Verification items for the finished model (mm, model axes). A direction names the side the tool comes from. Coordinates: 2 decimals unless noted, no trailing zeros. Write each loop counter-clockwise with the first axis right and the second up, starting at its lowest first coordinate (ties: lowest second). Pieces come first, ordered by that corner, then holes. Notation, with made-up numbers: (88.5, 30.5) -> (143.5, 30.5) arc R17 ccw to (143.5, 50.5) -> close; hole circle Ø7 at (85.25, -25). An arc over 180 degrees is marked (long way). Answer in a Markdown table with one row per item.
Autodesk Inventor part; units mm, degrees
ref_plane "YZ Plane" through (0, 0, 0) normal (1, 0, 0) x (0, 1, 0)
ref_plane "XZ Plane" through (0, 0, 0) normal (0, 1, 0) x (-1, 0, 0)
ref_plane "XY Plane" through (0, 0, 0) normal (0, 0, 1) x (1, 0, 0)
sketch "Sketch1" plane through (0, 0, 0) normal (0, 1, 0) x (-1, 0, 0)
  circle A0 centre (-30, -5.1319) radius 1.5
  arc A1 (-31.1155, 2.2846) -> (-30, -12.6319) centre (-30, -5.1319) ccw
  arc A2 (-30, -12.6319) -> (-31.1155, 2.2846) centre (-30, -5.1319) ccw construction
  circle A3 centre (-16.9706, -0.5878) radius 1.5
  circle A4 centre (16.9706, -0.5878) radius 1.5
  circle A5 centre (16.9706, -0.5878) radius 5 construction
  line L0 (-16.9706, 4.4122) -> (-31.1155, 2.2846)
  circle A6 centre (-16.9706, -0.5878) radius 5 construction
  circle A7 centre (-7.8058, -8.4213) radius 1.55
  line L1 (0, -8.4213) -> (-15.6117, -8.4213) construction
  circle A8 centre (0, 0) radius 1.55
  line L2 (-16.9706, 4.4122) -> (16.9706, 4.4122)
  line L3 (30, -12.6319) -> (-30, -12.6319)
  circle A9 centre (30, -5.1319) radius 1.5
  line L4 (0, 4.2106) -> (0, -4.2106) construction
  line L5 (0, -4.2106) -> (0, -12.6319) construction
  line L6 (0, -4.2106) -> (3.1574, -4.2106) construction
  line L7 (0, -8.4213) -> (15.6117, -8.4213) construction
  line L8 (16.9706, 4.4122) -> (31.1155, 2.2846)
  arc A10 (31.1155, 2.2846) -> (30, -12.6319) centre (30, -5.1319) ccw construction
  arc A11 (30, -12.6319) -> (31.1155, 2.2846) centre (30, -5.1319) ccw
  circle A12 centre (7.8058, -8.4213) radius 1.55
  point P0 (0, 0)
  point P1 (0, 0)
  dimension "d0" = 10
  dimension "d1" = 10
  dimension "d2" = 15
  dimension "d3" = 15
  dimension "d4" = 3.1
  dimension "d5" = 3.1
  dimension "d6" = 3.1
sketch "Sketch2" plane through (0, 0, 0) normal (0, 1, 0) x (-1, 0, 0)
  circle A0 centre (15, 9.8681) radius 3
  circle A1 centre (16.9706, -0.5878) radius 1.5
  arc A2 (3.1574, 6.6664) -> (-3.1574, 6.6664) centre (0, 4.2106) ccw
  line L0 (3.1574, 6.6664) -> (11.0366, -3.464)
  arc A3 (11.0366, -3.464) -> (13.9152, -6.7248) centre (38.6639, 18.024) ccw
  line L1 (13.9152, -6.7248) -> (21.1612, -13.9708)
  arc A4 (30.0072, 37.5736) -> (30.286, 34.6489) centre (32.7505, 36.3595) ccw
  arc A5 (35.8309, 43.8114) -> (30.0072, 37.5736) centre (41.895, 32.3124) ccw
  circle A6 centre (25.4558, 41.8386) radius 1.5
  circle A7 centre (30, 54.8681) radius 1.5
  circle A8 centre (16.9706, 50.3239) radius 1.5
  circle A9 centre (15, 39.8681) radius 3
  circle A10 centre (24.2029, 72.4055) radius 1.5
  line L2 (27.7949, 74.3102) -> (17.0958, 107.9924)
  arc A11 (17.0958, 107.9924) -> (14.6505, 110.5406) centre (13.2835, 106.7814) ccw
  circle A12 centre (13.2835, 106.7814) radius 1.5
  line L3 (14.6505, 110.5406) -> (2.0505, 115.1224)
  circle A13 centre (-24.2029, 72.4055) radius 1.5
  arc A14 (2.0505, 115.1224) -> (-2.0505, 115.1224) centre (0, 109.4837) ccw
  line L4 (-17.0958, 107.9924) -> (-27.7949, 74.3102)
  circle A15 centre (-13.2835, 106.7814) radius 1.5
  arc A16 (-14.6505, 110.5406) -> (-17.0958, 107.9924) centre (-13.2835, 106.7814) ccw
  line L5 (-2.0505, 115.1224) -> (-14.6505, 110.5406)
  line L6 (-25.5, 17.3681) -> (-25.5, 32.3681)
  line L7 (-28.5, 32.3681) -> (-28.5, 17.3681)
  line L8 (-31, 32.3681) -> (-31, 17.3681)
  arc A17 (-28.5, 17.3681) -> (-25.5, 17.3681) centre (-27, 17.3681) ccw
  arc A18 (-31, 17.3681) -> (-30.286, 15.0873) centre (-27, 17.3681) ccw
  arc A19 (-30.0072, 37.5736) -> (-35.8309, 43.8114) centre (-41.895, 32.3124) ccw
  arc A20 (-25.5, 32.3681) -> (-28.5, 32.3681) centre (-27, 32.3681) ccw
  arc A21 (-30.286, 34.6489) -> (-31, 32.3681) centre (-27, 32.3681) ccw
  arc A22 (-30.286, 34.6489) -> (-30.0072, 37.5736) centre (-32.7505, 36.3595) ccw
  circle A23 centre (-25.4558, 41.8386) radius 1.5
  circle A24 centre (-15, 39.8681) radius 3
  circle A25 centre (-16.9706, 50.3239) radius 1.5
  arc A26 (-30.0072, 12.1625) -> (-30.286, 15.0873) centre (-32.7505, 13.3766) ccw
  arc A27 (-35.8309, 5.9248) -> (-30.0072, 12.1625) centre (-41.895, 17.4238) ccw
  arc A28 (-35.8309, 5.9248) -> (-21.1612, -13.9708) centre (-30, -5.1319) ccw
  line L9 (-21.1612, -13.9708) -> (-13.9152, -6.7248)
  circle A29 centre (-15, 9.8681) radius 3
  circle A30 centre (-25.4558, 7.8975) radius 1.5
  circle A31 centre (-16.9706, -0.5878) radius 1.5
  circle A32 centre (-30, -5.1319) radius 1.5
  line L10 (-11.0366, -3.464) -> (-3.1574, 6.6664)
  arc A33 (-13.9152, -6.7248) -> (-11.0366, -3.464) centre (-38.6639, 18.024) ccw
  line L11 (31, 17.3681) -> (31, 32.3681)
  arc A34 (28.5, 32.3681) -> (25.5, 32.3681) centre (27, 32.3681) ccw
  line L12 (25.5, 32.3681) -> (25.5, 17.3681)
  line L13 (28.5, 17.3681) -> (28.5, 32.3681)
  arc A35 (31, 32.3681) -> (30.286, 34.6489) centre (27, 32.3681) ccw
  arc A36 (-34.9925, 66.3278) -> (-27.7949, 74.3102) centre (-40.1848, 78.2458) ccw
  arc A37 (-34.9925, 66.3278) -> (-35.8309, 43.8114) centre (-30, 54.8681) ccw
  circle A38 centre (-30, 54.8681) radius 1.5
  arc A39 (30.0072, 12.1625) -> (35.8309, 5.9248) centre (41.895, 17.4238) ccw
  circle A40 centre (30, -5.1319) radius 1.5
  arc A41 (21.1612, -13.9708) -> (35.8309, 5.9248) centre (30, -5.1319) ccw
  circle A42 centre (25.4558, 7.8975) radius 1.5
  arc A43 (25.5, 17.3681) -> (28.5, 17.3681) centre (27, 17.3681) ccw
  arc A44 (30.286, 15.0873) -> (30.0072, 12.1625) centre (32.7505, 13.3766) ccw
  arc A45 (30.286, 15.0873) -> (31, 17.3681) centre (27, 17.3681) ccw
  arc A46 (35.8309, 43.8114) -> (34.9925, 66.3278) centre (30, 54.8681) ccw
  arc A47 (27.7949, 74.3102) -> (34.9925, 66.3278) centre (40.1848, 78.2458) ccw
  circle A48 centre (-30, -5.1319) radius 1.5 construction
  point P0 (0, 0)
  point P1 (0, 109.4837)
sketch "Sketch3" plane through (0, 0, 0) normal (0, 1, 0) x (-1, 0, 0)
  arc A0 (3.1574, 6.6664) -> (-3.1574, 6.6664) centre (0, 4.2106) ccw
  line L0 (-11.0366, -3.464) -> (-3.1574, 6.6664)
  line L1 (3.1574, 6.6664) -> (11.0366, -3.464)
  arc A1 (11.0366, -3.464) -> (13.9152, -6.7248) centre (38.6639, 18.024) ccw
  arc A2 (-13.9152, -6.7248) -> (-11.0366, -3.464) centre (-38.6639, 18.024) ccw
  line L2 (-21.1612, -13.9708) -> (-13.9152, -6.7248)
  line L3 (13.9152, -6.7248) -> (21.1612, -13.9708)
  line L4 (30, -12.6319) -> (-30, -12.6319)
  circle A3 centre (-7.8058, -8.4213) radius 1.55 construction
  circle A4 centre (7.8058, -8.4213) radius 1.55 construction
  circle A5 centre (0, 0) radius 1.55
  circle A6 centre (-16.9706, -0.5878) radius 1.5 construction
  circle A7 centre (16.9706, -0.5878) radius 1.5 construction
  line L5 (-16.9706, -2.0878) -> (16.9706, -2.0878) construction
  line L6 (7.8058, -12.6319) -> (7.8058, -2.0878) construction
  line L7 (-7.8058, -12.6319) -> (-7.8058, -2.0878) construction
  circle A8 centre (-7.8058, -7.3599) radius 1.5
  circle A9 centre (7.8058, -7.3599) radius 1.5
  line L8 (-5.032, -12.6319) -> (-5.032, -2.0878) construction
  line L9 (-5.032, -7.3599) -> (-10.6888, -7.3599) construction
  point P0 (0, 0)
  point P1 (-19.8223, -12.6319)
  point P2 (19.8223, -12.6319)
  dimension "d38" = 3
  dimension "d39" = 3
  dimension "d42" = 10.5442
extrude "Extrusion1" add sketch "Sketch3" along normal blind 6 contours L1 A1 L3 L4 L2 A2 L0 A0 | A8 | A9
sketch "Sketch4" plane through (19.8223, 0, -12.6319) normal (0, 0, -1) x (-1, 0, 0)
  line L0 (0, 0) -> (39.6447, 0)
  line L1 (39.6447, 0) -> (39.6447, 6)
  line L2 (0, 6) -> (39.6447, 6)
  line L3 (0, 0) -> (0, 6)
  point P0 (19.8223, 0)
extrude "Extrusion2" add sketch "Sketch4" along normal blind 8.5
sketch "Sketch5" plane through (0, 0, 0) normal (0, -1, 0) x (1, 0, 0)
  line L0 (-19.8223, -21.1319) -> (19.8223, -21.1319)
  line L1 (19.8223, -21.1319) -> (19.8223, -13.6319)
  line L2 (19.8223, -12.6319) -> (19.8223, -21.1319)
  line L3 (19.8223, -13.6319) -> (-19.8223, -13.6319)
  line L4 (-19.8223, -12.6319) -> (-19.8223, -21.1319)
  line L5 (-19.8223, -13.6319) -> (-19.8223, -21.1319)
  line L6 (-19.8223, -21.1319) -> (19.8223, -21.1319)
  point P0 (0, 0)
  dimension "d11" = 7.5
extrude "Extrusion3" add sketch "Sketch5" along normal blind 7
sketch "Sketch6" plane through (19.8223, 6, -12.6319) normal (1, 0, 0) x (0, 0, -1)
  line L0 (0, -6) -> (0, 0) construction
  line L1 (0, -6) -> (0, -11.9599) construction
  line L2 (0, -11.9599) -> (3.918, -11.9599) construction
  circle A0 centre (3.918, -11.9599) radius 2.55
  circle A1 centre (3.918, -11.9599) radius 4.5
  line L3 (1, -6) -> (1, -13) construction
  line L4 (1, -6) -> (1, -7) construction
  line L5 (1, -7) -> (-0.2839, -10.3492)
  line L6 (1, -7) -> (1, -8.5343)
  line L7 (1, -6) -> (1, -13)
  point P0 (-12.6319, -6)
  dimension "d15" = 5.96
  dimension "d16" = 3.918
  dimension "d17" = 5.1
  dimension "d18" = 9
  dimension "d20" = 1
fillet "Fillet2" radius 1 1 edges at (0, 0, -13.6319)
extrude "Extrusion4" add sketch "Sketch6" against normal up to surface (39.6447 mm away) contours A1
extrude "Extrusion5" cut sketch "Sketch6" against normal up to surface (39.6447 mm away) contours A0
fillet "Fillet3" radius 3 1 edges at (0, -7, -21.1319)
extrude "Extrusion6" add sketch "Sketch6" against normal up to surface (39.6447 mm away) contours A1 L5 L6
sketch "Sketch7" plane through (0, 6, 0) normal (0, 1, 0) x (1, 0, 0)
  line L0 (-19.8223, 12.6319) -> (-13.9152, 6.7248)
  arc A0 (-11.0366, 3.464) -> (-13.9152, 6.7248) centre (-38.6639, -18.024) ccw
  line L1 (-11.0366, 3.464) -> (-3.1574, -6.6664)
  arc A1 (-3.1574, -6.6664) -> (3.1574, -6.6664) centre (0, -4.2106) ccw
  line L2 (3.1574, -6.6664) -> (11.0366, 3.464)
  arc A2 (13.9152, 6.7248) -> (11.0366, 3.464) centre (38.6639, -18.024) ccw
  line L3 (13.9152, 6.7248) -> (19.8223, 12.6319)
  line L4 (19.8223, 12.6319) -> (19.8223, 21.1319)
  line L5 (-19.8223, 21.1319) -> (19.8223, 21.1319)
  line L6 (-19.8223, 12.6319) -> (-19.8223, 21.1319)
  circle A3 centre (0, 0) radius 1.55
  point P0 (0, 0)
extrude "Extrusion7" add sketch "Sketch7" along normal blind 6
fillet "Fillet4" radius 8 1 edges at (0, 12, -21.1319)
sketch "Sketch8" plane through (0, 12, 0) normal (0, 1, 0) x (1, 0, 0)
  line L0 (0, 0) -> (0, 27.291) construction
  line L1 (-0.7613, 27.291) -> (-17.5, 27.291) construction
  line L2 (0.7613, 27.291) -> (17.5, 27.291) construction
  line L3 (-17.5, 27.291) -> (-17.5, 7.1815)
  line L4 (17.5, 27.291) -> (17.5, 7.1815)
  line L5 (17.5, 7.1815) -> (23.8846, 7.1815)
  line L6 (23.8846, 7.1815) -> (23.8846, 23.5209)
  line L7 (-17.5, 7.1815) -> (-22.9652, 7.1815)
  line L8 (-22.9652, 7.1815) -> (-22.9652, 23.5209)
  line L9 (-22.9652, 23.5209) -> (23.8846, 23.5209)
  point P0 (17.5, 23.5209)
  point P1 (-17.5, 23.5209)
  dimension "d34" = 35
extrude "Extrusion8" cut sketch "Sketch8" against normal through all
sketch "Sketch9" plane through (0, 0, 0) normal (0, -1, 0) x (1, 0, 0)
  circle A0 centre (0, 0) radius 1.55
  circle A1 centre (-16.9706, -0.5878) radius 1.5
  circle A2 centre (16.9706, -0.5878) radius 1.5
  line L0 (-16.9706, -2.0878) -> (16.9706, -2.0878)
  line L1 (16.9706, -2.0878) -> (16.9706, 15.9474)
  line L2 (16.9706, 15.9474) -> (-16.9706, 15.341)
  line L3 (-16.9706, 15.341) -> (-16.9706, -2.0878)
  point P0 (0, 0)
  point P1 (-16.9706, 0.9122)
  point P2 (16.9706, 0.9122)
extrude "Extrusion9" cut sketch "Sketch9" against normal up to surface (12 mm away) contours A1 L3 L2 L1 A2 L0
fillet "Fillet5" radius 8 2 edges at (-9.9662, 6, -2.0878) (9.9662, 6, -2.0878)
extrude "Extrusion10" cut sketch "Sketch3" along normal up to surface (12 mm away) contours A8 | A9
properties part number "prig to kauri conversion front link"
1. Sectioned sample at C-C, the plane x = 14.5. Record the cut outline in (y, z).
Findings below:
| item | result |
|---|---|
| outline | (-7, -20.93) arc R3 ccw to (-5.91, -21.13) -> (4, -21.13) arc R8 ccw to (12, -13.13) -> (12, -7.31) -> (0, -7.31) -> (0, -12.63) arc R1 cw to (-1, -13.63) -> (-4.35, -12.35) arc R4.5 ccw (long way) to start; hole circle Ø5.1 at (-5.96, -16.55) |
2. Access from +Z, -Z, +X, -X, +Y, -Y to the whole of each face (thin tool, end or side, straight path). Record for faces 1 (the face through (0.25, -5.19, -18.98)), 2 (the face through (0.25, -2.65, -13)).
Findings below:
| item | result |
|---|---|
| face 1 | +X, -X |
| face 2 | +Z, +X, -X |
3. Sectioned sample at B-B, the plane z = -18. Record the cut outline in (x, y).
Findings below:
| item | result |
|---|---|
| outline | (-17.5, -10.22) -> (17.5, -10.22) -> (17.5, -8.06) -> (-17.5, -8.06) -> close; (-17.5, -3.86) -> (17.5, -3.86) -> (17.5, 10.35) -> (-17.5, 10.35) -> close |
4. Sectioned sample at D-D, the plane x = 7. Count the separate pieces of the cut face and the enclosed holes in it, and give its area (3 significant figures).
Findings below:
| item | result |
|---|---|
| separate pieces | 2 |
| enclosed holes | 1 |
| area | 245 mm² |
5. Release check for a two-part mould opening along X. For faces 3 (the face through (17.5, 1, -16)), 4 (the face through (-13.04, 5.92, -5.82)), 5 (the face through (0.245, 9.594, -18.851)), 6 (the face through (6.42, 5.92, -6.79)) record: released by +X, released by -X, zero draft, split by the parting line, or undercut.
Findings below:
| item | result |
|---|---|
| face 3 | released by +X |
| face 4 | released by -X |
| face 5 | zero draft |
| face 6 | undercut |
6. Go/stop test with flat-tipped pins: pin 1 (1 mm diameter, centred on x = -3, y = 6.5, fed in from -Z); pin 2 (8.5 mm diameter, centred on x = -4.5, z = -5, fed in from -Y). Record where each tip stops, or that it passes through.
Findings below:
| item | result |
|---|---|
| pin 1 | stops at z = -20.88 |
| pin 2 | stops at y = 0 |
7. Sectioned sample at A-A, the plane y = -6.5. Record the cut outline in (x, z).
Findings below:
| item | result |
|---|---|
| outline | (-17.5, -21.07) -> (17.5, -21.07) -> (17.5, -19.04) -> (-17.5, -19.04) -> close; (-17.5, -14.06) -> (17.5, -14.06) -> (17.5, -12.08) -> (-17.5, -12.08) -> close |
8. Material ranges on probe 1 along X at (y, z) = (4.5, -6.25); probe 2 along Y at (x, z) = (15.5, -10); probe 3 along Y at (x, z) = (-12.5, -14.5), recorded low to high. Write a range as from..to.
Findings below:
| item | result |
|---|---|
| probe 1 | x = -13.45..-8.81, -6.8..6.8, 8.81..13.45 |
| probe 2 | y = 0..12 |
| probe 3 | y = -9.97..-7.48, -4.44..11.88 |
